```python
from build123d import *

# Parameters (mm, degrees)
PAD_DEPTH   = 16
FILLET_R    = 25
FILLET001_R = 25


with BuildPart() as part:
    # Sketch → Pad (new body)
    with BuildSketch(Plane.XZ):
        Polygon((0, 0), (0, 1550), (150, 1700), (331.507568, 1700), (362.76424, 1522.734604), (312.76424, 1522.734604), (258.518351, 1468.488715), (392.010101, 1028.284271), (590, 1000), (570, 860), (493.498457, 830), (450, 0), align=None)
    extrude(amount=PAD_DEPTH)

    # Fillet
    fillet_edges = [part.edges().sort_by_distance(p)[0] for p in [
        (362.76424, -8, 1522.734604),
        (331.507568, -8, 1700),
        (150, -8, 1700),
        (0, -8, 1550),
        (0, -8, 0),
        (450, -8, 0),
        (590, -8, 1000),
        (570, -8, 860),
    ]]
    fillet(fillet_edges, radius=FILLET_R)

    # Fillet001
    fillet001_edges = [part.edges().sort_by_distance(p)[0] for p in [
        (493.498457, -8, 830),
        (392.010101, -8, 1028.284271),
        (258.518351, -8, 1468.488715),
        (312.76424, -8, 1522.734604),
    ]]
    fillet(fillet001_edges, radius=FILLET001_R)


solid = part.part
```
Design review of the part built by this model. Coordinates are the model's own, in mm. A direction names the side the tool comes from. Coordinates: 2 decimals unless noted, no trailing zeros. Loops run counter-clockwise (first coordinate to the right, second up) from the corner with the lowest first, then second, coordinate; pieces in that order, holes last.
Q1. To check wall thickness, follow line 1 (X direction, y = -9.25, z = 785.5); line 2 (X direction, y = -11.5, z = 1422); line 3 (Z direction, x = 533, y = -10.5). State the ranges of each line that lie inside material, in increasing order.
Reported:
line 1: x = 0 to 491.17
line 2: x = 0 to 272.62
line 3: z = 845.49 to 1008.14
Q2. The part is to be moulded in two halves that separate along Z. For faces 1 (the face through (472.24, -7.89, 424.33)), 2 (the face through (287.53, -7.89, 1497.5)), 3 (the face through (232, -16, 862)), say which applies: +Z half, -Z half, draft (parallel to the pull), parting line (faces both ways), or undercut.
Reported:
face 1: -Z half
face 2: undercut
face 3: draft
Q3. We need section A-A on y = -9. State the section outline as (x, z) points.
Reported:
outline: (0, 25) arc R25 ccw to (25, 0) - (426.28, 0) arc R25 ccw to (451.24, 23.69) - (492.66, 813.91) arc R25 cw to (508.49, 835.88) - (556.44, 854.68) arc R25 ccw to (572.06, 874.42) - (586.46, 975.25) arc R25 ccw to (565.25, 1003.54) - (407.78, 1026.03) arc R25 cw to (387.39, 1043.53) - (262.87, 1454.15) arc R25 cw to (269.11, 1479.08) - (305.44, 1515.41) arc R25 cw to (323.12, 1522.73) - (332.97, 1522.73) arc R25 ccw to (357.59, 1552.08) - (335.15, 1679.34) arc R25 ccw to (310.53, 1700) - (160.36, 1700) arc R25 ccw to (142.68, 1692.68) - (7.32, 1557.32) arc R25 ccw to (0, 1539.64) - close
Q4. Tool access review of faces 4 (the face through (74, -8, 1624)), 5 (the face through (324.256, -7.888, 1251.712)): name each direction out of +Z, -Z, +X, -X, +Y, -Y from which nothing blocks a thin tool from reaching the whole face with its end or side.
Reported:
face 4: +Z, -X, +Y, -Y
face 5: +X, +Y, -Y
Q5. We need section C-C on z = 495. State the section outline as (x, y) points, and give its area (3 significant figures).
Reported:
outline: (0, -16) - (475.94, -16) - (475.94, 0) - (0, 0) - close
area: 7,620 mm2
Q6. We need section B-B on x = 65.5. State the section outline as (y, z) points, and give its area (3 significant figures).
Reported:
outline: (-16, 0) - (0, 0) - (0, 1615.5) - (-16, 1615.5) - close
area: 25,800 mm2
Q7. For pin 1 (1 mm diameter, centred on y = -9.5, z = 1179.5, fed in from +X); pin 2 (6 mm diameter, centred on x = 431, y = -2.5, fed in from -Z); pin 3 (1 mm diameter, centred on y = -8.5, z = 1108, fed in from +X); pin 4 (2 mm diameter, centred on x = 221.5, z = 870.5, fed in from +Y), all flat-tipped, find the tip position at first contact; note any pin that passes through.
Reported:
pin 1: stops at x = 346.31
pin 2: stops at z = 0.06
pin 3: stops at x = 367.99
pin 4: stops at y = 0
